The listing builds one solid part. Answer for the finished solid, in the listing's coordinates (mm). A direction names the side the tool comes from. Coordinates: 2 decimals unless noted, no trailing zeros. Order: outer loops, then holes, each group sorted by start corner. A loop starts at its lowest first (then second) coordinate and runs counter-clockwise, first axis right, second up.
from build123d import *

# Parameters (mm, degrees)
SKETCH1_R           = 1.6
BOSS_EXTRUDE1_DEPTH = 3
SKETCH2_W           = 10
SKETCH2_H           = 10
BOSS_EXTRUDE2_DEPTH = 42
CHAMFER1_SIZE       = 5
SKETCH3_R           = 2.1
CUT_EXTRUDE1_DEPTH  = 52
SKETCH4_R           = 2.65
CUT_EXTRUDE2_DEPTH  = 0.5
SKETCH5_W           = 6
SKETCH5_H           = 4.513236852
BOSS_EXTRUDE3_DEPTH = 14.15
SKETCH6_R           = 1.2
CUT_EXTRUDE3_DEPTH  = 6
SKETCH7_W           = 6
SKETCH7_H           = 10.018921585
BOSS_EXTRUDE4_DEPTH = 5
SKETCH8_W           = 6.018924213
SKETCH8_H           = 5.505684733
BOSS_EXTRUDE5_DEPTH = 2.15
SKETCH9_W           = 6
SKETCH9_H           = 3
BOSS_EXTRUDE6_DEPTH = 19.15
SKETCH10_R          = 1.2
CUT_EXTRUDE4_DEPTH  = 64.766604599
FILLET3_R           = 2
FILLET4_R           = 4.25
FILLET5_R           = 4.25
FILLET6_R           = 4.25
FILLET7_R           = 4.25
FILLET8_START       = 17.362615229
FILLET8_DEPTH       = 7.820980384
FILLET8_START_2     = 14.037603206
FILLET8_2_DEPTH     = 12.4500001
FILLET8_START_3     = 3
FILLET8_3_DEPTH     = 2
FILLET9_R           = 1


with BuildPart() as part:
    # Sketch1 → Boss-Extrude1 (new body)
    with BuildSketch(Plane(origin=(0, 0, 0), x_dir=(1, 0, 0), z_dir=(0, 1, 0))):
        Polygon((-6.512396694, 9.685950413), (1.487603306, 9.685950413), (26.487603306, 9.685950413), (26.487603306, -40.314049587), (1.487603306, -40.314049587), (-6.512396694, -40.314049587), align=None)
        with Locations(Location((-1.962396694, -35.764049587, 0), (0, 0, 270))):
            Circle(SKETCH1_R, mode=Mode.SUBTRACT)
        with Locations(Location((-1.962396694, 5.135950413, 0), (0, 0, 270))):
            Circle(SKETCH1_R, mode=Mode.SUBTRACT)
    extrude(amount=BOSS_EXTRUDE1_DEPTH)

    # Sketch2 → Boss-Extrude2 (add)
    with BuildSketch(Plane(origin=(0, 3, 0), x_dir=(1, 0, 0), z_dir=(0, 1, 0))):
        with Locations((21.487603306, -35.314049587)):
            Rectangle(SKETCH2_W, SKETCH2_H)
        with Locations((21.487603306, 4.685950413)):
            Rectangle(SKETCH2_W, SKETCH2_H)
    extrude(amount=BOSS_EXTRUDE2_DEPTH)

    # Chamfer1
    chamfer1_edges = [part.edges().sort_by_distance(p)[0] for p in [
        (21.487603306, 3, 30.314049587),
        (16.487603306, 3, 35.314049587),
        (16.487603306, 3, -4.685950413),
        (21.487603306, 3, 0.314049587),
    ]]
    chamfer(chamfer1_edges, length=CHAMFER1_SIZE)

    # Sketch3 → Cut-Extrude1 (cut)
    with BuildSketch(Plane(origin=(0, 45, 0), x_dir=(1, 0, 0), z_dir=(0, 1, 0))):
        with Locations(Location((22.537603306, -36.364049587, 0), (0, 0, 270))):
            Circle(SKETCH3_R)
        with Locations(Location((22.537603306, 5.735950413, 0), (0, 0, 270))):
            Circle(SKETCH3_R)
    extrude(amount=-CUT_EXTRUDE1_DEPTH, mode=Mode.SUBTRACT)

    # Sketch4 → Cut-Extrude2 (cut)
    with BuildSketch(Plane(origin=(0, 45, 0), x_dir=(1, 0, 0), z_dir=(0, 1, 0))):
        with Locations(Location((22.537603306, -36.364049587, 0), (0, 0, 270))):
            Circle(SKETCH4_R)
        with Locations(Location((22.537603306, 5.735950413, 0), (0, 0, 270))):
            Circle(SKETCH4_R)
    cut_extrude2 = extrude(amount=-CUT_EXTRUDE2_DEPTH, mode=Mode.SUBTRACT)

    # Mirror1: Cut-Extrude2 across plane
    add(cut_extrude2.mirror(Plane(origin=(0, 22.5, 0), x_dir=(0, 0, 1), z_dir=(0, -1, 0))), mode=Mode.SUBTRACT)

    # Sketch5 → Boss-Extrude3 (add)
    with BuildSketch(Plane(origin=(0, 0, -9.685950413), x_dir=(-1, 0, 0), z_dir=(0, 0, -1))):
        with Locations((-21.287603306, 33.943381574)):
            Rectangle(SKETCH5_W, SKETCH5_H)
    extrude(amount=BOSS_EXTRUDE3_DEPTH)

    # Sketch6 → Cut-Extrude3 (cut)
    with BuildSketch(Plane(origin=(24.287603306, 0, 0), x_dir=(0, 0, -1), z_dir=(1, 0, 0))):
        with Locations(Location((17.835950413, 34.5, 0), (0, 0, 90))):
            Circle(SKETCH6_R)
    extrude(amount=-CUT_EXTRUDE3_DEPTH, mode=Mode.SUBTRACT)

    # Sketch7 → Boss-Extrude4 (add)
    with BuildSketch(Plane(origin=(0, 0, -23.835950413), x_dir=(-1, 0, 0), z_dir=(0, 0, -1))):
        with Locations((-21.287603306, 36.696223941)):
            Rectangle(SKETCH7_W, SKETCH7_H)
    extrude(amount=BOSS_EXTRUDE4_DEPTH)

    # Sketch8 → Boss-Extrude5 (add)
    with BuildSketch(Plane(origin=(0, 0, -9.685950413), x_dir=(-1, 0, 0), z_dir=(0, 0, -1))):
        with Locations((-21.278141199, 38.952842367)):
            Rectangle(SKETCH8_W, SKETCH8_H)
    extrude(amount=BOSS_EXTRUDE5_DEPTH)

    # Sketch9 → Boss-Extrude6 (add)
    with BuildSketch(Plane(origin=(0, 0, -9.685950413), x_dir=(-1, 0, 0), z_dir=(0, 0, -1))):
        with Locations((-21.287603306, 1.5)):
            Rectangle(SKETCH9_W, SKETCH9_H)
    extrude(amount=BOSS_EXTRUDE6_DEPTH)

    # Sketch10 → Cut-Extrude4 (cut, through all)
    with BuildSketch(Plane(origin=(0, 41.705684733, 0), x_dir=(1, 0, 0), z_dir=(0, 1, 0))):
        with Locations(Location((21.287603306, 26.335950413, 0), (0, 0, 270))):
            Circle(SKETCH10_R)
    extrude(amount=-CUT_EXTRUDE4_DEPTH, mode=Mode.SUBTRACT)

    # Fillet3
    fillet3_edges = [part.edges().sort_by_distance(p)[0] for p in [
        (24.287603306, 36.696223941, -28.835950413),
        (18.287603306, 36.696223941, -28.835950413),
        (18.287603306, 1.5, -28.835950413),
        (24.287603306, 1.5, -28.835950413),
    ]]
    fillet(fillet3_edges, radius=FILLET3_R)

    # Fillet4
    # the kernel refuses this fillet: 4.25 mm, written as the material it adds along each edge
    with BuildSketch(Plane(origin=(24.287603306, 3, -9.685950413), x_dir=(0, 0, -1), z_dir=(0, -1, 0))) as fillet4_piece_1:
        with BuildLine():
            CenterArc((3.722902094, 4.25), FILLET4_R, 208.839189401, 61.160810599)
            Line((0, 2.2), (-0.074458042, 2.159))
            ThreePointArc((-0.074458042, 2.159), (-0.085, 1.1), (-0.085, 0))
            Line((-0.085, 0), (0, -0.085))
            Line((0, -0.085), (3.722902094, -0.085))
            Line((3.722902094, -0.085), (3.722902094, 0))
        make_face()
    extrude(amount=3)

    # Fillet5
    fillet5_edges = [part.edges().sort_by_distance(p)[0] for p in [
        (18.287603306, 1.5, -9.685950413),
    ]]
    fillet(fillet5_edges, radius=FILLET5_R)

    # Fillet6
    # the kernel refuses this fillet: 4.25 mm, written as the material it adds along each edge
    with BuildSketch(Plane(origin=(24.287603306, 31.686763148, -9.685950413), x_dir=(1, 0, 0), z_dir=(0, 1, 0))) as fillet6_piece_1_section:
        with BuildLine():
            CenterArc((4.25, 3.722902094), FILLET6_R, 180, 61.160810599)
            Line((0, 3.722902094), (-0.085, 3.722902094))
            Line((-0.085, 3.722902094), (-0.085, 0))
            Line((-0.085, 0), (0, -0.085))
            ThreePointArc((0, -0.085), (1.1, -0.085), (2.159, -0.074458042))
            Line((2.159, -0.074458042), (2.2, 0))
        make_face()
    fillet6_piece_1 = extrude(amount=10.018921585, mode=Mode.PRIVATE)
    fillet6_piece_1 = split(fillet6_piece_1, bisect_by=Plane(origin=(24.287603306, 31.686763148, -11.835950413), z_dir=(0, 0, 1)), keep=Keep.TOP, mode=Mode.PRIVATE)
    fillet6_piece_1 = split(fillet6_piece_1, bisect_by=Plane(origin=(24.287603306, 36.2, -9.685950413), z_dir=(0, -1, 0)), keep=Keep.TOP, mode=Mode.PRIVATE)
    add(fillet6_piece_1)
    with BuildSketch(Plane(origin=(24.287603306, 31.686763148, -9.685950413), x_dir=(1, 0, 0), z_dir=(0, 1, 0))) as fillet6_piece_2_section:
        with BuildLine():
            CenterArc((4.25, 3.722902094), FILLET6_R, 180, 61.160810599)
            Line((0, 3.722902094), (-0.085, 3.722902094))
            Line((-0.085, 3.722902094), (-0.085, 0))
            Line((-0.085, 0), (0, -0.085))
            ThreePointArc((0, -0.085), (1.1, -0.085), (2.159, -0.074458042))
            Line((2.159, -0.074458042), (2.2, 0))
        make_face()
    fillet6_piece_2 = extrude(amount=10.018921585, mode=Mode.PRIVATE)
    fillet6_piece_2 = split(fillet6_piece_2, bisect_by=Plane(origin=(24.287603306, 31.686763148, -11.835950413), z_dir=(0, 0, -1)), keep=Keep.TOP, mode=Mode.PRIVATE)
    fillet6_piece_2 = split(fillet6_piece_2, bisect_by=Plane(origin=(24.287603306, 36.2, -9.685950413), z_dir=(0, -1, 0)), keep=Keep.TOP, mode=Mode.PRIVATE)
    add(fillet6_piece_2)
    with BuildSketch(Plane(origin=(24.287603306, 31.686763148, -9.685950413), x_dir=(1, 0, 0), z_dir=(0, 1, 0))) as fillet6_piece_3_section:
        with BuildLine():
            CenterArc((4.25, 3.722902094), FILLET6_R, 180, 61.160810599)
            Line((0, 3.722902094), (-0.085, 3.722902094))
            Line((-0.085, 3.722902094), (-0.085, 0))
            Line((-0.085, 0), (0, -0.085))
            ThreePointArc((0, -0.085), (1.1, -0.085), (2.159, -0.074458042))
            Line((2.159, -0.074458042), (2.2, 0))
        make_face()
    fillet6_piece_3 = extrude(amount=10.018921585, mode=Mode.PRIVATE)
    fillet6_piece_3 = split(fillet6_piece_3, bisect_by=Plane(origin=(24.287603306, 31.686763148, -11.835950413), z_dir=(0, 0, 1)), keep=Keep.TOP, mode=Mode.PRIVATE)
    fillet6_piece_3 = split(fillet6_piece_3, bisect_by=Plane(origin=(24.287603306, 36.2, -9.685950413), z_dir=(0, 1, 0)), keep=Keep.TOP, mode=Mode.PRIVATE)
    add(fillet6_piece_3)

    # Fillet7
    # the kernel refuses this fillet: 4.25 mm, written as the material it adds along each edge
    with BuildSketch(Plane(origin=(18.287603306, 31.686763148, -9.685950413), x_dir=(0, 0, -1), z_dir=(0, 1, 0))) as fillet7_piece_1:
        with BuildLine():
            CenterArc((3.472751071, 4.25), FILLET7_R, 215.202683568, 54.797316432)
            Line((0, 1.8), (0, 0))
            Line((0, 0), (3.472751071, 0))
        make_face()
    extrude(amount=4.513236852)

    # Fillet8: read off the stored shape, not the designer's step
    # Fillet8 outline → Fillet8 (add)
    with BuildSketch(Plane.YZ.offset(FILLET8_START)):
        with BuildLine():
            ThreePointArc((3, -10.685950413), (3.292893219, -9.978843632), (4, -9.685950413))
            Line((4, -9.685950413), (3, -9.685950413))
            Line((3, -9.685950413), (3, -10.685950413))
        make_face()
    extrude(amount=FILLET8_DEPTH)

    # Fillet8 2 outline → Fillet8 2 (add)
    with BuildSketch(Plane.YZ.offset(FILLET8_START_2)):
        with BuildLine():
            ThreePointArc((3, -10.685950413), (3.292893219, -9.978843632), (4, -9.685950413))
            Line((4, -9.685950413), (3, -9.685950413))
            Line((3, -9.685950413), (3, -10.685950413))
        make_face()
    extrude(amount=FILLET8_2_DEPTH)

    # Fillet8 3 outline → Fillet8 3 (cut)
    with BuildSketch(Plane(origin=(0, 0, 0), x_dir=(1, 0, 0), z_dir=(0, 1, 0)).offset(FILLET8_START_3)):
        with BuildLine():
            ThreePointArc((25.274429362, 10.685950413), (25.834372953, 10.129363879), (26.487603306, 9.685950413))
            Line((26.487603306, 9.685950413), (26.487603306, 10.685950413))
            Line((26.487603306, 10.685950413), (25.274429362, 10.685950413))
        make_face()
        with BuildLine():
            Line((14.037603206, 10.685950413), (14.037603306, 9.685950413))
            ThreePointArc((14.037603306, 9.685950413), (15.495341279, 9.943770557), (16.776216093, 10.685950413))
            Line((16.776216093, 10.685950413), (14.037603206, 10.685950413))
        make_face()
    extrude(amount=FILLET8_3_DEPTH, mode=Mode.SUBTRACT)

    # Fillet9
    # the kernel refuses this fillet: 1 mm, written as the material it adds along each edge
    with BuildSketch(Plane(origin=(26.487603306, 31.686763148, -9.685950413), x_dir=(0, -1, 0), z_dir=(-1, 0, 0))) as fillet9_piece_1_section:
        with BuildLine():
            CenterArc((FILLET9_R, -FILLET9_R), FILLET9_R, 90, 90)
            Line((0, -FILLET9_R), (0, 0))
            Line((0, 0), (FILLET9_R, 0))
        make_face()
    fillet9_piece_1 = extrude(amount=10, mode=Mode.PRIVATE)
    fillet9_piece_1 = fillet9_piece_1 - Plane(origin=(14.037603306, 31.686763148, -13.158701484), x_dir=(0, 0, -1), z_dir=(0, -1, 0)) * Cylinder(4.25, 25, mode=Mode.PRIVATE)
    fillet9_piece_1 = fillet9_piece_1 - Plane(origin=(28.537603306, 31.686763148, -13.408852507), x_dir=(1, 0, 0), z_dir=(0, -1, 0)) * Cylinder(4.25, 25, mode=Mode.PRIVATE)
    add(fillet9_piece_1)


solid = part.part
(1) A tool of negligible diameter and unlimited length cuts with its end or side. For faces 5 (the flat face through (24.288, 1, -20)), 6 (the flat face through (21, 31.687, -20)), 7 (the flat face through (20.549, 5.465, 2.849)), 8 (the flat face through (21, 0.5, -4)), 9 (the flat face through (16.488, 26, 35)), from which of +Z, -Z, +X, -X, +Y, -Y can it reach the whole face along a straight path? Write none if from no direction.
(2) Find section B-B on y = 20. Determine the outline of the cut face in (x, z).
(3) Find the intervals of material crossed by probe 1 along X at (y, z) = (42.5, -5.5); probe 2 along Z at (x, y) = (23.5, 24); probe 3 along Z at (x, y) = (19.5, 34.5), in increasing order.
(4) Given pin 1 Ø2.5 at (y, z) = (2, -23) entering from -X; pin 2 Ø3 at (x, z) = (14.5, -13) entering from -Y; pin 3 Ø5 at (x, z) = (3.5, 29) entering from +Y; pin 4 Ø5 at (x, z) = (23, 26) entering from +Y, each flat-ended and moving along its own axis, determine where each tip first touches the part or whether it passes through.
(5) Find section A-A on y = 34.5. Determine the outline of the cut face in (x, z).
(6) Find section C-C on z = -4.5. Determine the outline of the cut face in (x, y), then the cut area to 3 significant figures.
(7) Find section D-D on y = 40. Determine the outline of the cut face in (x, z).
(8) The mould has two halves that part along Z. Classify faces 1 (the flat face through (7, 3, 15)), 2 (the flat face through (18, 15, -9.686)), 3 (the cylindrical face through (-2.58, 1.48, -3.66)), 4 (the flat face through (20, 45, 34)): pulls with the +Z half, pulls with the -Z half, needs draft (parallel to the pull), parting line crosses it, or undercut.
Resolved:
1. face 5: -Z, +X, +Y, -Y
1. face 6: -Z, +X, -X
1. face 7: +X, -X, +Y
1. face 8: -Y
1. face 9: +Z, -Z, -X, +Y
2. outline: (16.49, -9.69) - (26.49, -9.69) - (26.49, 0.31) - (16.49, 0.31) - close; (16.49, 30.31) - (26.49, 30.31) - (26.49, 40.31) - (16.49, 40.31) - close; hole circle Ø4.2 at (22.54, -5.74); hole circle Ø4.2 at (22.54, 36.36)
3. probe 1: x = 16.49 to 20.45, 24.62 to 26.49
3. probe 2: z = -9.69 to -7.6, -3.87 to 0.31, 30.31 to 34.5, 38.23 to 40.31
3. probe 3: z = -28.67 to -19.04, -16.64 to 0.31, 30.31 to 40.31
4. pin 1: stops at x = 18.29
4. pin 2: passes through
4. pin 3: stops at y = 3
4. pin 4: stops at y = 6.19
5. outline: (16.49, -9.69) arc R4.25 cw to (18.29, -13.16) - (18.29, -16.64) - (24.29, -16.64) - (24.29, -13.41) arc R4.25 cw to (26.49, -9.69) - (26.49, 0.31) - (16.49, 0.31) - close; (16.49, 30.31) - (26.49, 30.31) - (26.49, 40.31) - (16.49, 40.31) - close; (18.29, -26.84) arc R2 ccw to (20.29, -28.84) - (22.29, -28.84) arc R2 ccw to (24.29, -26.84) - (24.29, -19.04) - (18.29, -19.04) - close; hole circle Ø2.4 at (21.29, -26.34); hole circle Ø4.2 at (22.54, -5.74); hole circle Ø4.2 at (22.54, 36.36)
6. outline: (-6.51, 0) - (-3.43, 0) - (-3.43, 3) - (-6.51, 3) - close; (-0.49, 0) - (20.19, 0) - (20.19, 0.5) - (20.84, 0.5) - (20.84, 44.5) - (20.19, 44.5) - (20.19, 45) - (16.49, 45) - (16.49, 8) - (11.49, 3) - (-0.49, 3) - close; (24.24, 0.5) - (24.88, 0.5) - (24.88, 0) - (26.49, 0) - (26.49, 45) - (24.88, 45) - (24.88, 44.5) - (24.24, 44.5) - close
6. area: 369 mm2
7. outline: (16.49, -9.69) - (18.27, -9.69) - (18.27, -11.84) - (24.59, -11.84) arc R4.25 cw to (26.49, -9.69) - (26.49, 0.31) - (16.49, 0.31) - close; (16.49, 30.31) - (26.49, 30.31) - (26.49, 40.31) - (16.49, 40.31) - close; (18.29, -26.84) arc R2 ccw to (20.29, -28.84) - (22.29, -28.84) arc R2 ccw to (24.29, -26.84) - (24.29, -23.84) - (18.29, -23.84) - close; hole circle Ø2.4 at (21.29, -26.34); hole circle Ø4.2 at (22.54, -5.74); hole circle Ø4.2 at (22.54, 36.36)
8. face 1: undercut
8. face 2: pulls with the -Z half
8. face 3: undercut
8. face 4: needs draft
